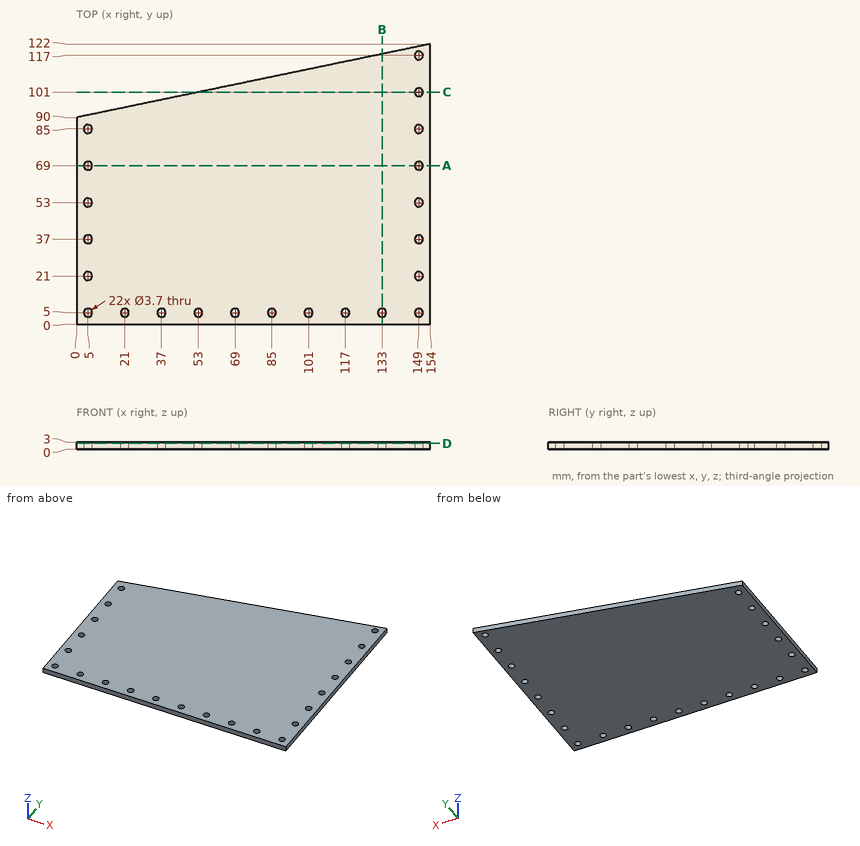
Input: dimensioned drawing with shaded views. Units: mm. Origin: part minimum x, y, z. Coordinates: 2 decimals unless noted, no trailing zeros. Loops run counter-clockwise (first coordinate to the right, second up) from the corner with the lowest first, then second, coordinate; pieces in that order, holes last. Notation, with made-up numbers: (-6.5, -22.75) -> (0.5, -22.75) arc R25 cw to (0.5, -3.75) -> close; hole circle Ø8 at (6, 8.5). An arc over 180 degrees is marked (long way). Use a Markdown table: item, result. Add a question column.
(1) Section query C-C, the plane y = 101. Return loops of the section in (x, z).
(2) Section query D-D, the plane z = 2.55. State how many separate pieces and enclosed holes the cut face has, plus the area to 3 significant figures.
(3) Section query B-B, the plane x = 133. Return loops of the section in (y, z), plus the area to 3 significant figures.
(4) Line query: line 1 along X through (y, z) = (52, 1.1); line 2 along Y through (x, z) = (69, 1.4); line 3 along Y through (x, z) = (102, 2.4). Output: solid intervals per line, ascending.
(5) Section query A-A, the plane y = 69. Return loops of the section in (x, z).
Answer:
| question | item | result |
|---|---|---|
| 1 | outline | (52.94, 0) -> (147.15, 0) -> (147.15, 3) -> (52.94, 3) -> close; (150.85, 0) -> (154, 0) -> (154, 3) -> (150.85, 3) -> close |
| 2 | separate pieces | 1 |
| 2 | enclosed holes | 22 |
| 2 | area | 16,100 mm^2 |
| 3 | outline | (0, 0) -> (3.15, 0) -> (3.15, 3) -> (0, 3) -> close; (6.85, 0) -> (117.64, 0) -> (117.64, 3) -> (6.85, 3) -> close |
| 3 | area | 342 mm^2 |
| 4 | line 1 | x = 0 to 3.44, 6.56 to 147.44, 150.56 to 154 |
| 4 | line 2 | y = 0 to 3.15, 6.85 to 104.34 |
| 4 | line 3 | y = 0 to 3.44, 6.56 to 111.19 |
| 5 | outline | (0, 0) -> (3.15, 0) -> (3.15, 3) -> (0, 3) -> close; (6.85, 0) -> (147.15, 0) -> (147.15, 3) -> (6.85, 3) -> close; (150.85, 0) -> (154, 0) -> (154, 3) -> (150.85, 3) -> close |
